Input: dimensioned drawing with shaded views. Units: mm. Origin: part minimum x, y, z. Give positions to 0.01 mm unless a question says otherwise; leave off trailing zeros. Loops run counter-clockwise (first coordinate to the right, second up) from the corner with the lowest first, then second, coordinate; pieces in that order, holes last.
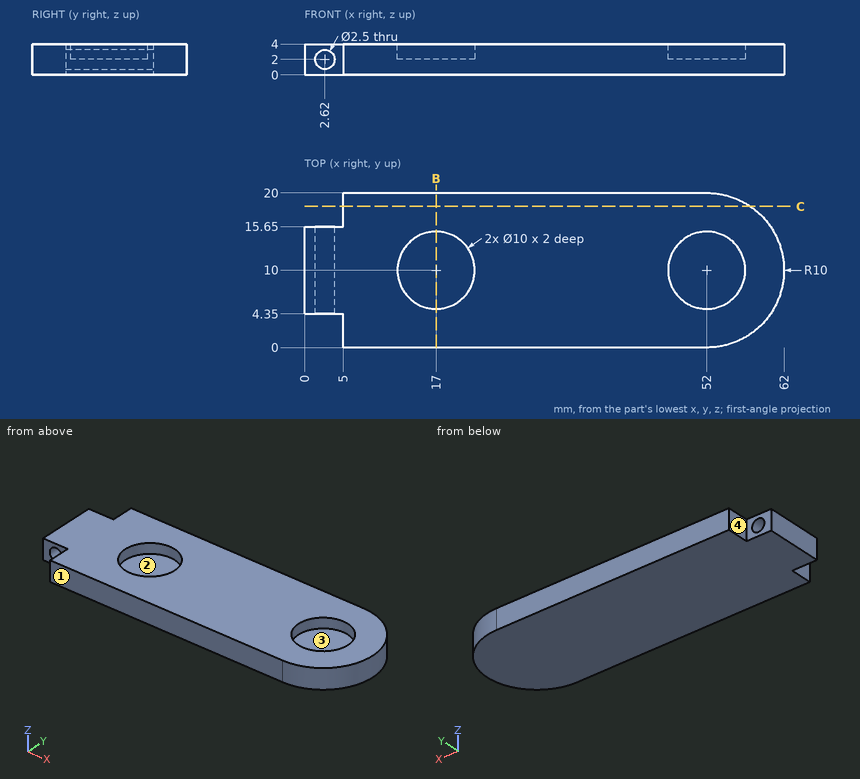
Item 1: Pin query (flat end, axial travel): pin 1 (1 mm diameter, centred on y = 17.5, z = 2.5, fed in from -X); pin 2 (2 mm diameter, centred on x = 2.5, z = 2.5, fed in from -Y). Return the tip coordinate at first contact, or that it passes through.
Values follow:
pin 1: stops at x = 5
pin 2: stops at y = 4.35
Item 2: Draft query along X for the marked faces 1, 2, 3 and 4. Return one class per face: +X half, -X half, draft (parallel to the pull), parting line (faces both ways), or undercut.
Values follow:
face 1: draft
face 2: undercut
face 3: undercut
face 4: -X half
Item 3: Ray query, probe 1 along X at (y, z) = (12.75, 2.95) (1 decimal); probe 2 along Y at (x, z) = (17, 2.65); probe 3 along Z at (x, y) = (48, 9). Return the intervals inside material, ascending.
Values follow:
probe 1: x = 0 to 1.8, 3.4 to 12.8, 21.2 to 47.8, 56.2 to 61.6
probe 2: y = 0 to 5, 15 to 20
probe 3: z = 0 to 2
Item 4: Section query C-C on y = 18.25. Return loops of the section in (x, z).
Values follow:
outline: (5, 0) - (57.65, 0) - (57.65, 4) - (5, 4) - close
Item 5: Section query B-B on x = 17. Return loops of the section in (y, z).
Values follow:
outline: (0, 0) - (20, 0) - (20, 4) - (15, 4) - (15, 2) - (5, 2) - (5, 4) - (0, 4) - close
